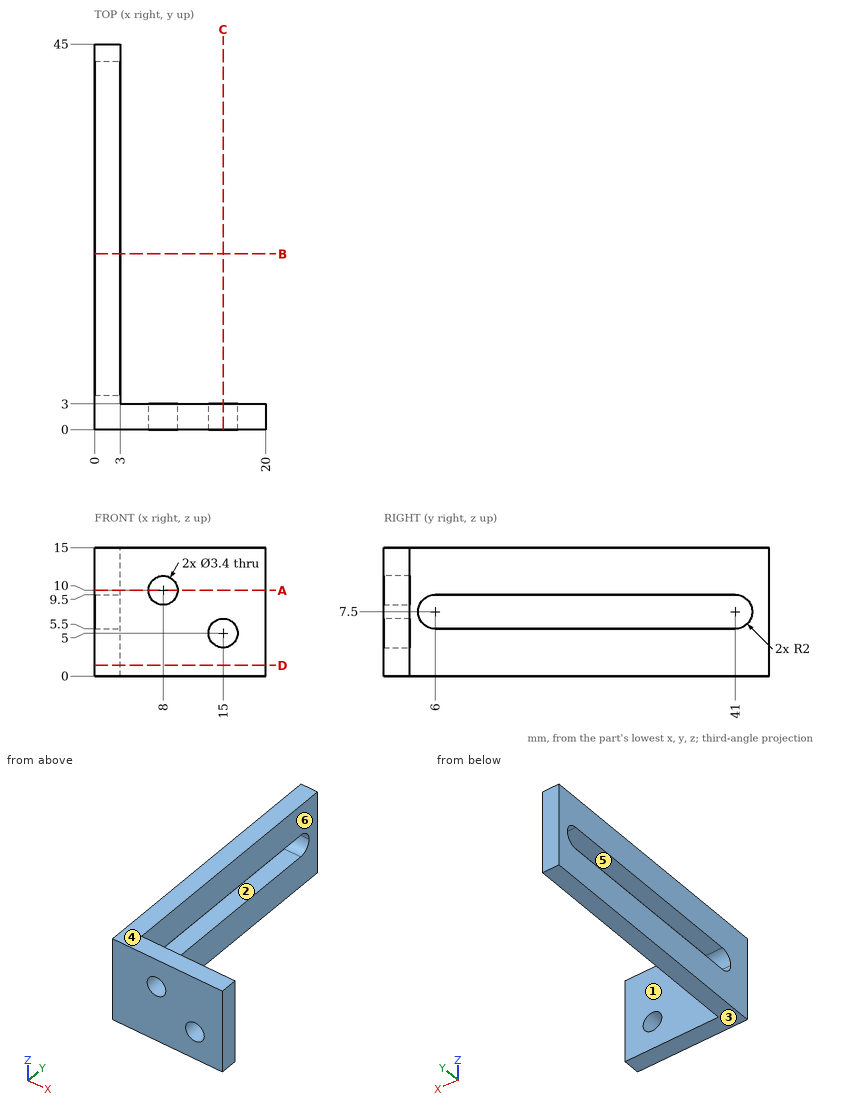
The figure shows three views and two pictorial views of one solid part (mm, origin at its lowest corner). Answer the questions. A direction names the side the tool comes from. Round coordinates to 2 decimals unless told otherwise and drop trailing zeros. Loops run counter-clockwise (first coordinate to the right, second up) from the corner with the lowest first, then second, coordinate; pieces in that order, holes last. Notation, with made-up numbers: M 41.5,79.25 L 89.5,79.25 A18 cw 89.5,114.25 Z; hole C 19.5,2.5 d11. An arc over 180 degrees is marked long. Write each question's results on one line, items separated by ' | '. Start each with the question number.
1) Straight lines are drawn through the part: probe 1 along X at (y, z) = (2.4, 10); probe 2 along X at (y, z) = (15, 3.25). For each, find the intervals that lie inside material, in ascending order.
2) Each of these flat-tipped pins is pushed along its axis until it touches: pin 1 (4.5 mm diameter, centred on x = 15, z = 5, fed in from +Y); pin 2 (6 mm diameter, centred on y = 20.5, z = 7.5, fed in from +X); pin 3 (5 mm diameter, centred on y = 8.5, z = 5.5, fed in from -X). Where does it stop, or does it pass through?
3) Determine the mould class of the marked faces 1, 2 and 3 for opening direction Y: pulls with the +Y half, pulls with the -Y half, needs draft (parallel to the pull), parting line crosses it, or undercut.
4) Which of the six approach directions +Z, -Z, +X, -X, +Y, -Y give full straight-line access (tool end or side, diameter ignored) to the marked faces 4, 5 and 6?
5) Find section B-B on y = 20.5. Write down the section's boundary in (x, z), plus the area to 3 significant figures.
6) Find section D-D on z = 1.25. Write down the section's boundary in (x, y).
7) Find section C-C on x = 15. Write down the section's boundary in (y, z), plus the area to 3 significant figures.
8) Find section A-A on z = 10. Write down the section's boundary in (x, y), plus the area to 3 significant figures.
Final values:
1) probe 1: 0 to 6.3, 9.7 to 20 | probe 2: 0 to 3
2) pin 1: y = 3 | pin 2: x = 3 | pin 3: x = 0
3) face 1: pulls with the +Y half | face 2: undercut | face 3: needs draft
4) face 4: +Z, +X, -X, +Y, -Y | face 5: +X, -X | face 6: +Z, -Z, +X, +Y
5) outline: M 0,0 L 3,0 L 3,5.5 L 0,5.5 Z; M 0,9.5 L 3,9.5 L 3,15 L 0,15 Z | area: 33.0 mm²
6) outline: M 0,0 L 20,0 L 20,3 L 3,3 L 3,45 L 0,45 Z
7) outline: M 0,0 L 3,0 L 3,3.3 L 0,3.3 Z; M 0,6.7 L 3,6.7 L 3,15 L 0,15 Z | area: 34.8 mm²
8) outline: M 0,0 L 6.3,0 L 6.3,3 L 3,3 L 3,45 L 0,45 Z; M 9.7,0 L 20,0 L 20,3 L 9.7,3 Z | area: 176 mm²
